```python
from build123d import *

# Parameters (mm, degrees)
F0_R     = 4.1965730186
F1_DEPTH = 2.54
F2_DEPTH = 1.27
F3_SIZE  = 1.26999
F4_SIZE  = 2.53999


# Not quite as in the source:
# - a fillet or chamfer is up to 0.001 mm smaller than in the source, because OpenCascade refuses the exact size


with BuildPart() as f1:
    # F0 (on Top) → F1 (new body, symmetric)
    with BuildSketch(Plane.XY):
        with BuildLine():
            ThreePointArc((0, 49.7234201631), (-9.6606227132, 42.7095239111), (-5.9829372688, 31.3518392168))
            Line((-5.9829372688, 31.3518392168), (-1.8358110683, 27.2047130163))
            Line((-1.8358110683, 27.2047130163), (-1.8358110683, 17.501438998))
            Line((-1.8358110683, 17.501438998), (0, 16.2159902493))
            Line((0, 16.2159902493), (1.8358110683, 17.501438998))
            Line((1.8358110683, 17.501438998), (1.8358110683, 27.2047130163))
            Line((1.8358110683, 27.2047130163), (5.9829372688, 31.3518392168))
            ThreePointArc((5.9829372688, 31.3518392168), (9.6606227132, 42.7095239111), (0, 49.7234201631))
        make_face()
        with Locations((0, 39.5634201631)):
            Circle(F0_R, mode=Mode.SUBTRACT)
    extrude(amount=F1_DEPTH, both=True)

    # F0 (on Top) → F2 (join, symmetric)
    with BuildSketch(Plane.XY):
        Polygon((-1.8358110683, 27.2047130163), (-5.9829372688, 31.3518392168), (-5.9829372688, 16.1118392168), (0, 11.9225414406), (5.9829372688, 16.1118392168), (5.9829372688, 31.3518392168), (1.8358110683, 27.2047130163), (1.8358110683, 17.501438998), (0, 16.2159902493), (-1.8358110683, 17.501438998), align=None)
    extrude(amount=F2_DEPTH, both=True)

    # F3 (size 1.27 in the source; OpenCascade refuses exactly that, so slightly less here)
    f3_edges = [f1.edges().sort_by_distance(p)[0] for p in [
        (0.917906, 16.858715, 1.27),
        (-0.917906, 16.858715, 1.27),
        (1.835811, 22.353076, 1.27),
        (-1.835811, 22.353076, 1.27),
        (5.982937, 23.731839, 1.27),
        (-5.982937, 23.731839, 1.27),
        (-2.991469, 14.01719, 1.27),
        (2.991469, 14.01719, 1.27),
        (2.991469, 14.01719, -1.27),
        (5.982937, 23.731839, -1.27),
        (0.917906, 16.858715, -1.27),
        (1.835811, 22.353076, -1.27),
        (-0.917906, 16.858715, -1.27),
        (-1.835811, 22.353076, -1.27),
        (-5.982937, 23.731839, -1.27),
        (-2.991469, 14.01719, -1.27),
    ]]
    chamfer(f3_edges, length=F3_SIZE)

    # F4 (size 2.54 in the source; OpenCascade refuses exactly that, so slightly less here)
    f4_edges = [f1.edges().sort_by_distance(p)[0] for p in [
        (-4.196573, 39.56342, 2.54),
        (-4.196573, 39.56342, -2.54),
    ]]
    chamfer(f4_edges, length=F4_SIZE)


solid = f1.part
```
The model under review builds one solid part; all positions refer to its coordinate system, in mm. A direction names the side the tool comes from. Give positions to 0.01 mm unless a question says otherwise; leave off trailing zeros. Loops run counter-clockwise (first coordinate to the right, second up) from the corner with the lowest first, then second, coordinate; pieces in that order, holes last. Notation, with made-up numbers: (8, -32) - (25, -32) arc R27 ccw to (25, -13) - close; hole circle Ø2 at (79, -23). An arc over 180 degrees is marked (long way). Answer as a JSON object with one key per item and string values.
Q1. Add section B-B on z = 0.75. State the section outline as (x, y) points, plus the area to 3 significant figures.
Worked out:
{"outline": "(-5.98, 31.35) - (-5.23, 30.6) - (-5.23, 16.5) - (0, 12.84) - (5.23, 16.5) - (5.23, 30.6) - (5.98, 31.35) arc R10.16 ccw (long way) to start; hole circle Ø9.89 at (0, 39.56)", "area": "407 mm^2"}
Q2. To check wall thickness, follow line 1 along Z through (x, y) = (-3.5, 16); line 2 along X through (y, z) = (43.5, -2.3); line 3 along Y through (x, z) = (3.75, 0.75). State the ranges of each line that lie inside material, in increasing order.
Worked out:
{"line 1": "z = -1.27 to 1.27", "line 2": "x = -9.37 to -5.17, 5.17 to 9.37", "line 3": "y = 15.46 to 36.34, 42.79 to 49.01"}
Q3. Insertion check: pin 1 (3 mm diameter, centred on y = 27, z = -1, fed in from -X); pin 2 (2 mm diameter, centred on y = 30, z = 0, fed in from +X). Each pin has a flat end and moves straight along its axis. Give the tip position at first contact, or say it passes through.
Worked out:
{"pin 1": "stops at x = -5.98", "pin 2": "stops at x = 5.98"}
Q4. Mouldability with a two-part tool opening along Y and no side actions: class faces 4 (the flat face through (5.357, 23.625, -0.626)), 5 (the conical face through (2.01, 35.7, -0.16)), 6 (the flat face through (1.205, 16.296, -1.914)) as +Y half, -Y half, draft (parallel to the pull), parting line (faces both ways), or undercut.
Worked out:
{"face 4": "draft", "face 5": "undercut", "face 6": "-Y half"}
Q5. For faces 1 (the flat face through (4.34, 29.71, -1.82)), 2 (the flat face through (-2.462, 22.576, -1.914)), 3 (the flat face through (-4, 21, -1.27)), list the 3-axis set-ups (+Z, -Z, +X, -X, +Y, -Y) from which the entire face can be reached by the end or side of a thin tool; tool diameter is ignored.
Worked out:
{"face 1": "-Z, +X, -Y", "face 2": "-Z, -X, -Y", "face 3": "-Z, -Y"}
Q6. Add section D-D on x = 8.25. State the section outline as (y, z) points.
Worked out:
{"outline": "(33.63, -2.54) - (45.49, -2.54) - (45.49, 2.54) - (33.63, 2.54) - close"}
